Can you work these out from the model? Positions are in its coordinate system, mm. A direction names the side the tool comes from. Round coordinates to 2 decimals unless told otherwise and drop trailing zeros. Write each loop counter-clockwise with the first axis right and the second up, starting at its lowest first coordinate (ties: lowest second). Pieces come first, ordered by that corner, then holes.
Q1. For faces 1 (the flat face through (21, -2, 4)), 2 (the flat face through (3, -2, 4)), 3 (the flat face through (10, -12, 0)), 4 (the flat face through (12, -5, 9)), which set-ups out of +Z, -Z, +X, -X, +Y, -Y let a thin tool reach every point of the face, with its end or its side?
Q2. If we section it at B-B (y = -10.5): Please give me the cut outline in (x, z).
Q3. We'd pull the mould along Y, two halves only. Please class faces 5 (the flat face through (12, 0, 2)), 6 (the flat face through (12, -20, 9)), 7 (the flat face through (12, -13, 4)), 8 (the flat face through (20, -12, -2)): +Y half, -Y half, draft (parallel to the pull), parting line (faces both ways), or undercut.
Q4. Please list where these lines run through material, in increasing order: line 1 along Z through (x, y) = (3.75, -16); line 2 along Y through (x, z) = (12.5, 6.75); line 3 along X through (y, z) = (-16, -2.75).
Q5. If we section it at A-A (x = 12): Please give me the cut outline in (y, z), plus the area to 3 significant figures.
Q6. I'm going to push flat-ended pins straight in: pin 1 Ø10 at (x, y) = (12.5, -18) entering from +Z; pin 2 Ø2.5 at (x, y) = (2, -22) entering from +Z; pin 3 Ø5 at (x, y) = (17, -20) entering from +Z. Where does each tip first touch, or does it pass through?
Q7. If we section it at C-C (z = 8.5): Please give me the cut outline in (x, y).
Q8. If we section it at D-D (x = 4.75): Please give me the cut outline in (y, z), plus the area to 3 significant figures.
from build123d import *

# Parameters (mm, degrees)
PAD_DEPTH         = 25
SKETCH001_W       = 15
SKETCH001_H       = 16.832567
POCKET_DEPTH      = 0.001
POCKET_DEPTH_BACK = -24.001


with BuildPart() as part:
    # Sketch → Pad (new body)
    with BuildSketch(Plane.XZ):
        with BuildLine():
            Line((0, 0), (20, 0))
            Line((20, 0), (20, -4))
            Line((20, -4), (0, -4))
            Line((0, -4), (0, -8.041044))
            Line((0, -8.041044), (24, -8.041044))
            Line((24, -8.041044), (24, 4))
            Line((24, 4), (17.988441, 4))
            Line((15.983215, 14.366061), (17.988441, 4))
            ThreePointArc((15.983215, 14.366061), (11.968793, 17.999878), (8.011559, 14.303867))
            Line((8.011559, 14.303867), (6.011559, 4))
            Line((6.011559, 4), (0, 4))
            Line((0, 4), (0, 0))
        make_face()
    extrude(amount=PAD_DEPTH)

    # Sketch001 → Pocket (cut, two sides)
    with BuildSketch(Plane.YZ) as pocket_sk:
        with Locations((-12.5, 12.416283)):
            Rectangle(SKETCH001_W, SKETCH001_H)
    extrude(amount=-POCKET_DEPTH, mode=Mode.SUBTRACT)
    extrude(pocket_sk.sketch, amount=-POCKET_DEPTH_BACK, mode=Mode.SUBTRACT)


solid = part.part
A:
1. face 1: +Z, +X, +Y, -Y
1. face 2: +Z, -X, +Y, -Y
1. face 3: -X, +Y, -Y
1. face 4: +Z, +X, -X
2. outline: (0, -8.04) - (24, -8.04) - (24, 4) - (0, 4) - (0, 0) - (20, 0) - (20, -4) - (0, -4) - close
3. face 5: +Y half
3. face 6: undercut
3. face 7: undercut
3. face 8: draft
4. line 1: z = -8.04 to -4, 0 to 4
4. line 2: y = -25 to -20, -5 to 0
4. line 3: x = 20 to 24
5. outline: (-25, -8.04) - (0, -8.04) - (0, -4) - (-25, -4) - close; (-25, 0) - (0, 0) - (0, 18) - (-5, 18) - (-5, 4) - (-20, 4) - (-20, 18) - (-25, 18) - close
5. area: 341 mm2
6. pin 1: stops at z = 18
6. pin 2: stops at z = 4
6. pin 3: stops at z = 17.12
7. outline: (6.89, -25) - (17.12, -25) - (17.12, -20) - (6.89, -20) - close; (6.89, -5) - (17.12, -5) - (17.12, 0) - (6.89, 0) - close
8. outline: (-25, -8.04) - (0, -8.04) - (0, -4) - (-25, -4) - close; (-25, 0) - (0, 0) - (0, 4) - (-25, 4) - close
8. area: 201 mm2
